Autodesk Inventor part; units mm, degrees
ref_plane "YZ Plane" through (0, 0, 0) normal (1, 0, 0) x (0, 1, 0)
ref_plane "XZ Plane" through (0, 0, 0) normal (0, 1, 0) x (-1, 0, 0)
ref_plane "XY Plane" through (0, 0, 0) normal (0, 0, 1) x (1, 0, 0)
sketch "Sketch3" plane through (0, 0, 0) normal (0, 1, 0) x (-1, 0, 0)
  line L0 (37.5, 4.7) -> (-37.5, 4.7)
  line L1 (-37.5, 4.7) -> (-37.5, -4.7)
  line L2 (-37.5, -4.7) -> (37.5, -4.7)
  line L3 (37.5, -4.7) -> (37.5, 4.7)
  line L4 (37.5, 4.7) -> (-37.5, -4.7) construction
  line L5 (-37.5, 4.7) -> (37.5, -4.7) construction
  point P0 (0, 0)
  dimension "d0" = 75
  dimension "d1" = 9.4
extrude "Extrusion1" add sketch "Sketch3" along normal blind 7.5
sketch "Sketch4" plane through (0, 7.5, 0) normal (0, 1, 0) x (1, 0, 0)
  line L0 (-37.5, 4.7) -> (-37.5, -4.7)
  line L1 (-37.5, 0) -> (37.5, 0)
  line L2 (37.5, -4.7) -> (37.5, 4.7)
  line L3 (37.5, 4.7) -> (-37.5, 4.7)
  line L4 (0, 4.7) -> (0, -4.7)
  line L5 (-37.5, -4.7) -> (37.5, -4.7)
  line L6 (-35.2, 3.45) -> (-34.8, 3.45)
  line L7 (-34.8, 3.45) -> (-34.8, 4.05)
  line L8 (-34.8, 4.05) -> (-35.2, 4.05)
  line L9 (-35.2, 4.05) -> (-35.2, 3.45)
  line L10 (-35.2, 3.45) -> (-34.8, 4.05) construction
  line L11 (-34.8, 3.45) -> (-35.2, 4.05) construction
  line L12 (-35.2, -3.45) -> (-34.8, -3.45)
  line L13 (-34.8, -3.45) -> (-34.8, -4.05)
  line L14 (-34.8, -4.05) -> (-35.2, -4.05)
  line L15 (-35.2, -4.05) -> (-35.2, -3.45)
  line L16 (-35.2, -3.45) -> (-34.8, -4.05) construction
  line L17 (-34.8, -3.45) -> (-35.2, -4.05) construction
  line L18 (35.2, 3.45) -> (34.8, 3.45)
  line L19 (34.8, 3.45) -> (34.8, 4.05)
  line L20 (34.8, 4.05) -> (35.2, 4.05)
  line L21 (35.2, 4.05) -> (35.2, 3.45)
  line L22 (35.2, 3.45) -> (34.8, 4.05) construction
  line L23 (34.8, 3.45) -> (35.2, 4.05) construction
  line L24 (35.2, -3.45) -> (34.8, -3.45)
  line L25 (34.8, -3.45) -> (34.8, -4.05)
  line L26 (34.8, -4.05) -> (35.2, -4.05)
  line L27 (35.2, -4.05) -> (35.2, -3.45)
  line L28 (35.2, -3.45) -> (34.8, -4.05) construction
  line L29 (34.8, -3.45) -> (35.2, -4.05) construction
  point P0 (0, 0)
  point P1 (-35, 3.75)
  point P2 (-35, -3.75)
  point P3 (35, 3.75)
  point P4 (35, -3.75)
  dimension "d7" = 0.6
  dimension "d8" = 0.4
  dimension "d9" = 7.5
  dimension "d10" = 70
extrude "Extrusion2" add sketch "Sketch4" along normal blind 3.5 contours L9 L8 L7 L6 | L12 L13 L14 L15 | L18 L19 L20 L21 | L27 L26 L25 L24
sketch "Sketch5" plane through (0, 0, 0) normal (0, -1, 0) x (1, 0, 0)
  line L0 (-33.3, -1) -> (33.3, -1)
  line L1 (33.3, -1) -> (33.3, 1)
  line L2 (33.3, 1) -> (-33.3, 1)
  line L3 (-33.3, 1) -> (-33.3, -1)
  line L4 (-33.3, -1) -> (33.3, 1) construction
  line L5 (33.3, -1) -> (-33.3, 1) construction
  point P0 (0, 0)
  dimension "d13" = 66.6
  dimension "d14" = 2
extrude "Extrusion3" cut sketch "Sketch5" against normal blind 5
sketch "Sketch6" plane through (0, 0, 0) normal (0, -1, 0) x (1, 0, 0)
  circle A0 centre (-35.5, 0) radius 1
  line L0 (37.5, -4.7) -> (-37.5, -4.7)
  line L1 (0, -4.7) -> (0, 4.7)
  line L2 (-37.5, 4.7) -> (37.5, 4.7)
  circle A1 centre (35.5, 0) radius 1
  point P0 (0, 0)
  point P1 (0, 0)
  dimension "d17" = 2
  dimension "d18" = 71
extrude "Extrusion4" cut sketch "Sketch6" against normal blind 5
thread "Thread1"
thread "Thread2"
chamfer "Chamfer1" distance 0.2 angle 45 8 edges at (-37.5, 3.75, -4.7) (-37.5, 3.75, 4.7) (37.5, 3.75, -4.7) (37.5, 3.75, 4.7) (0, 0, -4.7) (37.5, 0, 0) (0, 0, 4.7) (-37.5, 0, 0)
chamfer "Chamfer2" distance 0.1 angle 45 32 edges at (-34.8, 9.25, -3.45) (-35.2, 9.25, -3.45) (-34.8, 9.25, -4.05) (-35.2, 9.25, -4.05) (-35.2, 11, -3.75) (-34.8, 11, -3.75) (-35, 11, -4.05) (-35, 11, -3.45) (-34.8, 9.25, 4.05) (-34.8, 11, 3.75) (-35, 11, 4.05) (-35.2, 11, 3.75) (-35.2, 9.25, 4.05) (-34.8, 9.25, 3.45) (-35, 11, 3.45) (-35.2, 9.25, 3.45) (34.8, 11, 3.75) (35, 11, 4.05) (35.2, 11, 3.75) (34.8, 9.25, 4.05) (35.2, 9.25, 4.05) (35, 11, 3.45) (34.8, 9.25, 3.45) (35.2, 9.25, 3.45) (34.8, 9.25, -3.45) (35, 11, -3.45) (35.2, 9.25, -3.45) (34.8, 11, -3.75) (34.8, 9.25, -4.05) (35.2, 11, -3.75) (35.2, 9.25, -4.05) (35, 11, -4.05)
Could you check a few things on this model? Use its own coordinates, in mm. A direction names the side the tool comes from. Give positions to 0.01 mm unless a question says otherwise; leave off trailing zeros. Order: outer loops, then holes, each group sorted by start corner. A loop starts at its lowest first (then second) coordinate and runs counter-clockwise, first axis right, second up. Notation, with made-up numbers: M 88.5,59.25 L 118.5,59.25 A18 cw 118.5,83.25 Z; hole C 12.25,53.25 d5. An arc over 180 degrees is marked long. One line per question, with ' | ' between items.
1. We'd pull the mould along Z, two halves only. Please class faces 1 (the face through (-1, 4, 4.7)), 2 (the face through (36.454, 2.465, 0.3)), 3 (the face through (1, 4, -4.7)): +Z half, -Z half, draft (parallel to the pull), parting line (faces both ways), or undercut.
Results:
face 1: +Z half | face 2: undercut | face 3: -Z half
2. I want a section at B-B (z = 0). List the corners of the cut face in (x, y) for me, and give its area (3 significant figures).
Results:
outline: M -37.5,0.2 L -37.3,0 L -36.5,0 L -36.5,5 L -34.5,5 L -34.5,0 L -33.3,0 L -33.3,5 L 33.3,5 L 33.3,0 L 34.5,0 L 34.5,5 L 36.5,5 L 36.5,0 L 37.3,0 L 37.5,0.2 L 37.5,7.5 L -37.5,7.5 Z | area: 209 mm²
3. I'm going to push flat-ended pins straight in: pin 1 (4 mm diameter, centred on x = 8.5, z = 1, fed in from -Y); pin 2 (5 mm diameter, centred on x = -2.5, z = 2, fed in from +Y); pin 3 (0.6 mm diameter, centred on x = 11.5, z = 0, fed in from -Y). Where does each tip first touch, or does it pass through?
Results:
pin 1: y = 0 | pin 2: y = 7.5 | pin 3: y = 5
4. I want a section at C-C (x = -25.5). List the corners of the cut face in (y, z) for me.
Results:
outline: M 0,-4.5 L 0.2,-4.7 L 7.5,-4.7 L 7.5,4.7 L 0.2,4.7 L 0,4.5 L 0,1 L 5,1 L 5,-1 L 0,-1 Z
5. If I drill on line 1 (Z direction, x = -25, y = 1); line 2 (Y direction, x = -31, z = 0.5); line 3 (Y direction, x = 7.5, z = 2), over which ranges is the centre line in solid material (lowest first)?
Results:
line 1: -4.7 to -1, 1 to 4.7 | line 2: 5 to 7.5 | line 3: 0 to 7.5
6. I want a section at A-A (y = 1.5). List the corners of the cut face in (x, z) for me.
Results:
outline: M -37.5,-4.5 L -37.3,-4.7 L 37.3,-4.7 L 37.5,-4.5 L 37.5,4.5 L 37.3,4.7 L -37.3,4.7 L -37.5,4.5 Z; hole C -35.5,0 d2; hole M -33.3,-1 L 33.3,-1 L 33.3,1 L -33.3,1 Z; hole C 35.5,0 d2
7. For faces 4 (the face through (0, 2, -1)), 5 (the face through (1, 0, 2)), which set-ups out of +Z, -Z, +X, -X, +Y, -Y let a thin tool reach every point of the face, with its end or its side?
Results:
face 4: -Y | face 5: +Z, -Z, +X, -X, -Y
